Autodesk Inventor part; units mm, degrees
ref_plane "YZ Plane" through (0, 0, 0) normal (1, 0, 0) x (0, 1, 0)
ref_plane "XZ Plane" through (0, 0, 0) normal (0, 1, 0) x (-1, 0, 0)
ref_plane "XY Plane" through (0, 0, 0) normal (0, 0, 1) x (1, 0, 0)
sketch "スケッチ12" plane through (0, 0, 0) normal (0, 0, 1) x (1, 0, 0)
  line L0 (0, 0) -> (54, 0)
  line L1 (54, 0) -> (54, 37)
  line L2 (54, 37) -> (0, 37)
  line L3 (0, 37) -> (0, 0)
  dimension "d76" = 54
  dimension "d77" = 37
extrude "押し出し7" add sketch "スケッチ12" along normal blind 20
sketch "スケッチ14" plane through (0, 37, 0) normal (0, 1, 0) x (1, 0, 0)
  line L0 (54, 0) -> (54, -20)
  line L1 (54, 0) -> (0, 0)
  line L2 (0, 0) -> (0, -20)
  point P0 (2.7, -5)
  point P1 (2.7, -15)
  point P2 (51.3, -5)
  point P3 (51.3, -15)
  dimension "d80" = 48.6
  dimension "d81" = 10
  dimension "d82" = 10
  dimension "d83" = 2.7
  dimension "d84" = 5
  dimension "d85" = 5
  dimension "d86" = 2.7
  dimension "d87" = 2.7
hole "穴3" at (2.7, 37, 5) at (2.7, 37, 15) at (51.3, 37, 5) at (51.3, 37, 15) direction (0, -1, 0) diameter 3.9 end through all
sketch "スケッチ15" plane through (0, 0, 20) normal (0, 0, 1) x (1, 0, 0)
  line L0 (0, 0) -> (6.55, 0)
  line L1 (6.55, 0) -> (6.55, 26.8)
  line L2 (6.55, 26.8) -> (0, 26.8)
  line L3 (0, 26.8) -> (0, 0)
  line L4 (54, 0) -> (54, 37)
  line L5 (54, 0) -> (47.45, 0)
  line L6 (47.45, 0) -> (47.45, 26.8)
  line L7 (47.45, 26.8) -> (54, 26.8)
  line L8 (54, 26.8) -> (54, 0)
  line L9 (54, 37) -> (0, 37)
  line L10 (0, 37) -> (6.55, 37)
  line L11 (6.55, 37) -> (6.55, 30)
  line L12 (6.55, 30) -> (0, 30)
  line L13 (0, 30) -> (0, 37)
  line L14 (54, 37) -> (47.45, 37)
  line L15 (47.45, 37) -> (47.45, 30)
  line L16 (47.45, 30) -> (54, 30)
  line L17 (54, 30) -> (54, 37)
  dimension "d100" = 26.8
  dimension "d101" = 6.55
  dimension "d102" = 40.9
  dimension "d103" = 7
extrude "押し出し8" cut sketch "スケッチ15" against normal blind 20
sketch "スケッチ16" plane through (6.55, 37, 0) normal (0, 1, 0) x (1, 0, 0)
  line L0 (47.45, -20) -> (47.45, 0)
  line L1 (47.45, -10) -> (-12.7368, -10)
  line L2 (-6.55, -20) -> (-6.55, 0)
  circle A0 centre (10.4, -10) radius 2.5
  circle A1 centre (44.75, -15) radius 1.95
  dimension "d106" = 5
  dimension "d107" = 34.35
extrude "押し出し9" add sketch "スケッチ16" along normal blind 5.7 contours A0 L1 | L1 A0
properties part number "servo"
Design review of the part built by this model. Coordinates are the model's own, in mm. A direction names the side the tool comes from. Give positions to 0.01 mm unless a question says otherwise; leave off trailing zeros. Write each loop counter-clockwise with the first axis right and the second up, starting at its lowest first coordinate (ties: lowest second). Pieces come first, ordered by that corner, then holes.
(1) Clearance check with flat-ended pins moving along their axes: pin 1 Ø2.5 at (x, z) = (2.7, 5) entering from -Y; pin 2 Ø10 at (x, y) = (32.5, 18) entering from -Z; pin 3 Ø3.5 at (y, z) = (33.5, 12.5) entering from -X; pin 4 Ø3.5 at (x, z) = (2.5, 13.5) entering from -Y. State where each tip first meets the part, or that it passes through.
Checked values:
pin 1: passes through
pin 2: stops at z = 0
pin 3: stops at x = 6.55
pin 4: stops at y = 26.8
(2) Add section C-C (z = 1.5). Give the boundary of the cut face in (x, y), and give its area (3 significant figures).
Checked values:
outline: (0, 26.8) - (6.55, 26.8) - (6.55, 0) - (47.45, 0) - (47.45, 26.8) - (54, 26.8) - (54, 30) - (47.45, 30) - (47.45, 37) - (6.55, 37) - (6.55, 30) - (0, 30) - close
area: 1,560 mm2
(3) Add section D-D (x = 16.95). Give the boundary of the cut face in (y, z), and give its area (4 significant figures).
Checked values:
outline: (0, 0) - (37, 0) - (37, 7.5) - (42.7, 7.5) - (42.7, 12.5) - (37, 12.5) - (37, 20) - (0, 20) - close
area: 768.5 mm2
(4) Tool access review of faces 1 (the face through (47.45, 34, 10)), 2 (the face through (16.41, 39.81, 7.56)), 3 (the face through (3, 30, 10)), 4 (the face through (47.45, 13, 10)), 5 (the face through (3, 26.8, 10)): name each direction out of +Z, -Z, +X, -X, +Y, -Y from which nothing blocks a thin tool from reaching the whole face with its end or side.
Checked values:
face 1: +Z, -Z, +X, +Y
face 2: +Y
face 3: +Z, -Z, -X, +Y
face 4: +Z, -Z, +X, -Y
face 5: +Z, -Z, -X, -Y
(5) Wall thickness on line 1 along Z through (x, y) = (51.3, 28); line 2 along X through (y, z) = (27.85, 5); line 3 along X through (y, z) = (22, 1.25): over which ranges is each line inside the solid? List them lowest first.
Checked values:
line 1: z = 0 to 3.05, 6.95 to 13.05, 16.95 to 20
line 2: x = 0 to 0.75, 4.65 to 49.35, 53.25 to 54
line 3: x = 6.55 to 47.45
(6) Add section B-B (x = 2.7). Give the boundary of the cut face in (y, z), and give its area (3 significant figures).
Checked values:
outline: (26.8, 0) - (30, 0) - (30, 3.05) - (26.8, 3.05) - close; (26.8, 6.95) - (30, 6.95) - (30, 13.05) - (26.8, 13.05) - close; (26.8, 16.95) - (30, 16.95) - (30, 20) - (26.8, 20) - close
area: 39.0 mm2
(7) Mouldability with a two-part tool opening along X and no side actions: class faces 6 (the face through (51, 30, 10)), 7 (the face through (2.614, 28.378, 13.052)), 8 (the face through (6.55, 34, 10)) as +X half, -X half, draft (parallel to the pull), parting line (faces both ways), or undercut.
Checked values:
face 6: draft
face 7: undercut
face 8: -X half
(8) Add section A-A (z = 15). Give the boundary of the cut face in (x, y), and give its area (3 significant figures).
Checked values:
outline: (0, 26.8) - (0.75, 26.8) - (0.75, 30) - (0, 30) - close; (4.65, 26.8) - (6.55, 26.8) - (6.55, 0) - (47.45, 0) - (47.45, 26.8) - (49.35, 26.8) - (49.35, 30) - (47.45, 30) - (47.45, 37) - (6.55, 37) - (6.55, 30) - (4.65, 30) - close; (53.25, 26.8) - (54, 26.8) - (54, 30) - (53.25, 30) - close
area: 1,530 mm2
